Design review of the part shown in the three views and the two pictorial views. Dimensions are in mm from the part's minimum x, y and z. Coordinates: 2 decimals unless noted, no trailing zeros. Order: outer loops, then holes, each group sorted by start corner. A loop starts at its lowest first (then second) coordinate and runs counter-clockwise, first axis right, second up. Notation, with made-up numbers: (47.5, -3.5) -> (64.5, -3.5) arc R17 cw to (64.5, 26.5) -> close; hole circle Ø7 at (-30.5, 87.5). An arc over 180 degrees is marked (long way). Answer as a JSON object with one key per item and string values. Group by question number.
1) Draft analysis for pull direction Z (two halves, no side actions). For the marked faces 1, 2, 3 and 4, state which applies: +Z half, -Z half, draft (parallel to the pull), parting line (faces both ways), or undercut.
2) For pin 1 (2 mm diameter, centred on y = 2, z = 4, fed in from -X); pin 2 (1.8 mm diameter, centred on x = 3, y = 3, fed in from +Z), all flat-tipped, find the tip position at first contact; note any pin that passes through.
3) Add section C-C, the plane x = 1.3. Write out the cut boundary in (y, z), then the cut area to 3 significant figures.
4) Add section A-A, the plane x = 3. Write out the cut boundary in (y, z), then the cut area to 3 significant figures.
5) Wall thickness on L1, parallel to Z at x = 3, y = 0.8: over which ranges is the line inside the solid? List them lowest first.
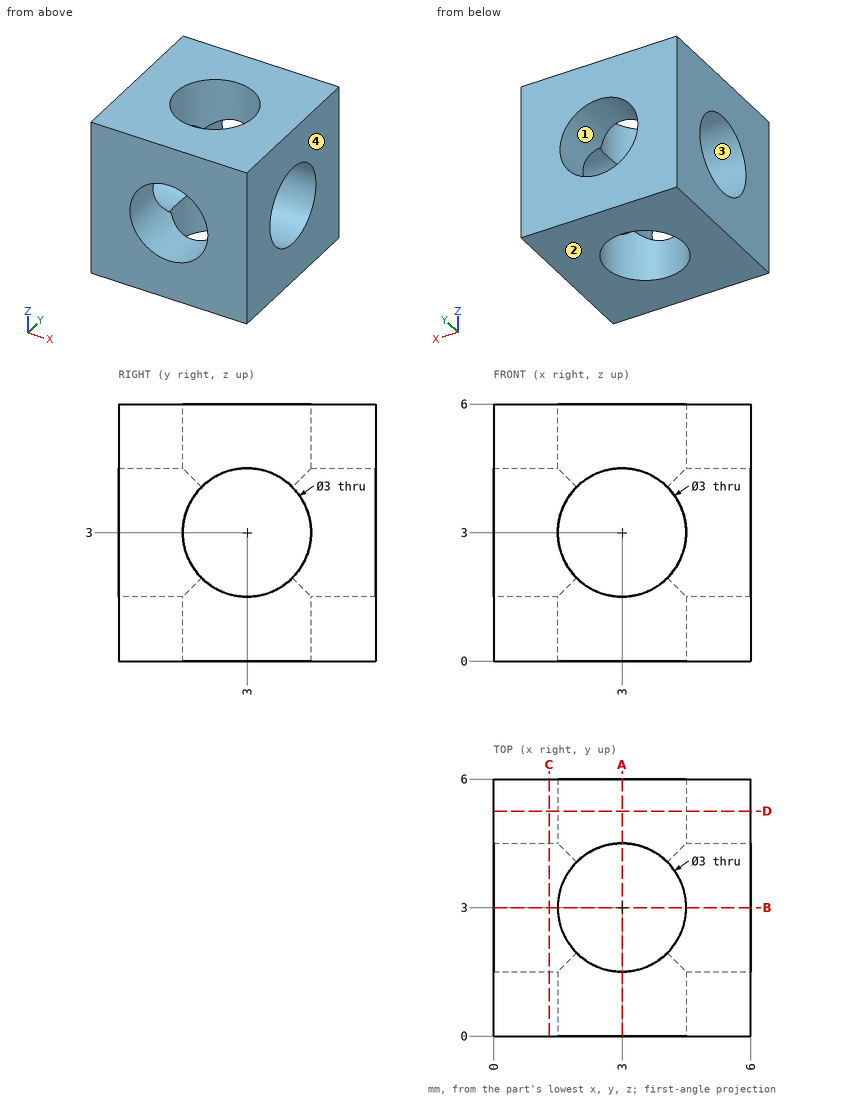
Output values:
{
 "1": {"face 1": "undercut", "face 2": "-Z half", "face 3": "undercut", "face 4": "draft"},
 "2": {"pin 1": "stops at x = 0", "pin 2": "passes through"},
 "3": {"outline": "(0, 0) -> (6, 0) -> (6, 6) -> (0, 6) -> close; hole circle Ø3 at (3, 3)", "area": "28.9 mm²"},
 "4": {"outline": "(0, 0) -> (1.5, 0) -> (1.5, 1.5) -> (0, 1.5) -> close; (0, 4.5) -> (1.5, 4.5) -> (1.5, 6) -> (0, 6) -> close; (4.5, 0) -> (6, 0) -> (6, 1.5) -> (4.5, 1.5) -> close; (4.5, 4.5) -> (6, 4.5) -> (6, 6) -> (4.5, 6) -> close", "area": "9.00 mm²"},
 "5": {"L1": "z = 0 to 1.5, 4.5 to 6"}
}
